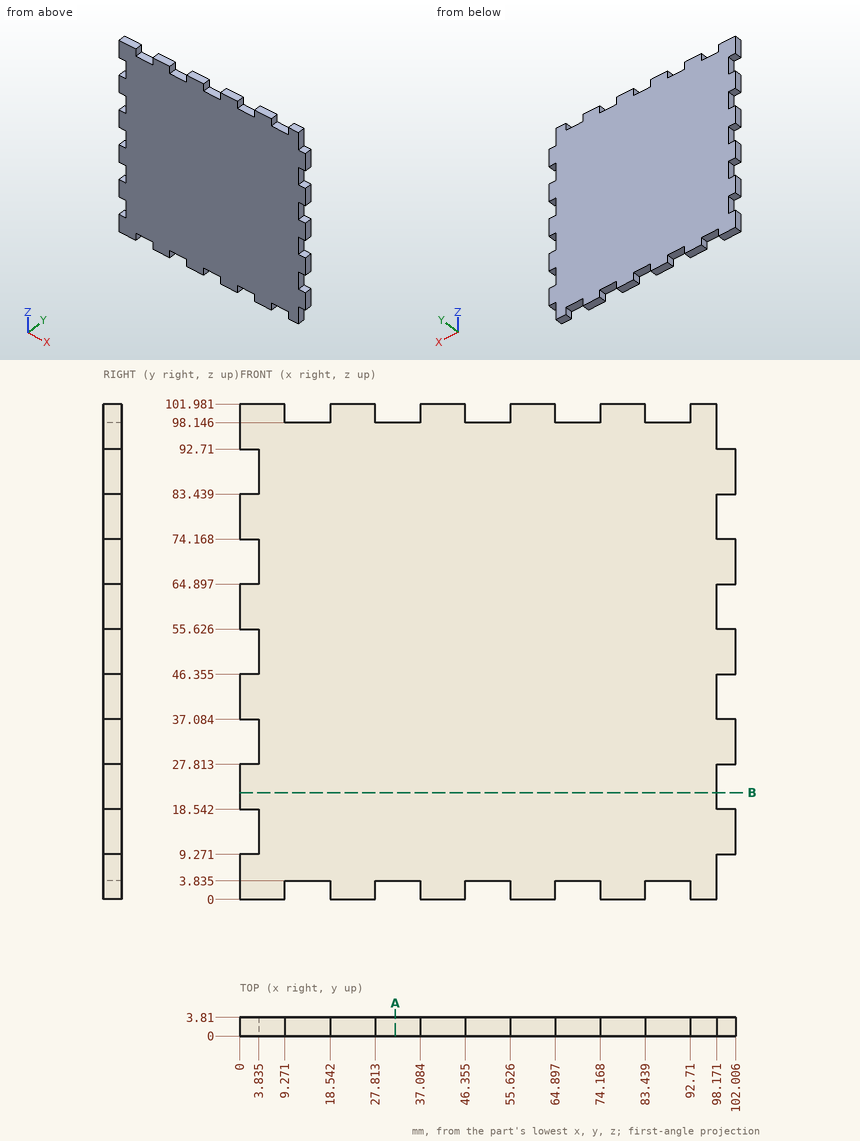
The figure shows three views and two pictorial views of one solid part (mm, origin at its lowest corner). Answer the questions. Coordinates: 2 decimals unless noted, no trailing zeros. Loops run counter-clockwise (first coordinate to the right, second up) from the corner with the lowest first, then second, coordinate; pieces in that order, holes last. Notation, with made-up numbers: (-10.75, 75.5) -> (25.25, 75.5) arc R19 cw to (25.25, 111.5) -> close; hole circle Ø4 at (80, 67). An arc over 180 degrees is marked (long way). Return JSON: item names as keys, results as strings. Group by question number.
(1) A cutting plane is placed at A-A on x = 32. Write down the section's boundary in (y, z) (1 decimal), and give its area (3 significant figures).
(2) Given pin 1 Ø1.9 at (y, z) = (2, 99.5) entering from +X; pin 2 Ø1.1 at (x, y) = (101, 2.5) entering from +Z; pin 3 Ø1.1 at (x, y) = (86, 1.5) entering from +Z, each flat-ended and moving along its own axis, determine where each tip first touches the part or whether it passes through.
(3) A cutting plane is placed at B-B on z = 22. Write down the section's boundary in (x, y).
(4) Find the intervals of material crossed by probe 1 along X at (y, z) = (2.15, 56.5); probe 2 along Z at (x, y) = (72, 3.1) (1 decimal); probe 3 along X at (y, z) = (3.65, 66) (1 decimal), in increasing order. Write a range as from..to.
The answers:
{
 "1": {"outline": "(0, 3.8) -> (3.8, 3.8) -> (3.8, 98.1) -> (0, 98.1) -> close", "area": "359 mm^2"},
 "2": {"pin 1": "stops at x = 98.17", "pin 2": "stops at z = 92.71", "pin 3": "stops at z = 98.15"},
 "3": {"outline": "(0, 0) -> (98.17, 0) -> (98.17, 3.81) -> (0, 3.81) -> close"},
 "4": {"probe 1": "x = 0..98.17", "probe 2": "z = 3.8..98.1", "probe 3": "x = 3.8..102"}
}
